Here's how the part is built. I have some questions about the finished solid (model axes, mm). Face numbers are marked on the shaded views. A direction names the side the tool comes from. Round coordinates to 2 decimals unless told otherwise and drop trailing zeros. Order: outer loops, then holes, each group sorted by start corner. A loop starts at its lowest first (then second) coordinate and runs counter-clockwise, first axis right, second up. Notation, with made-up numbers: (-6.75, -6.5) - (41.25, -6.5) arc R21 ccw to (41.25, 17.5) - close; hole circle Ø4 at (30, 83.5). An arc over 180 degrees is marked (long way). One line per item, written item: value.
Autodesk Inventor part; units mm, degrees
ref_plane "YZ Plane" through (0, 0, 0) normal (1, 0, 0) x (0, 1, 0)
ref_plane "XZ Plane" through (0, 0, 0) normal (0, 1, 0) x (-1, 0, 0)
ref_plane "XY Plane" through (0, 0, 0) normal (0, 0, 1) x (1, 0, 0)
sketch "Sketch1" plane through (0, 0, 0) normal (0, 0, 1) x (1, 0, 0)
  line L0 (0, 0) -> (8.89, 0)
  line L1 (8.89, 0) -> (8.89, 12.7)
  line L2 (8.89, 12.7) -> (0, 12.7)
  line L3 (0, 12.7) -> (0, 0)
  circle A0 centre (7.62, 1.27) radius 0.635
  circle A1 centre (1.27, 1.27) radius 0.635
  point P0 (4.445, 4.445)
  dimension "d0" = 8.89
  dimension "d1" = 12.7
  dimension "d18" = 1.27
  dimension "d19" = 1.27
  dimension "d20" = 1.27
  dimension "d21" = 1.27
  dimension "d22" = 1.27
  dimension "d23" = 1.27
  dimension "d26" = 4.445
extrude "Extrusion1" add sketch "Sketch1" along normal blind 2.54 contours L3 L2 L1 L0 | A0 | A1
sketch "Sketch2" plane through (0, 0, 2.54) normal (0, 0, 1) x (1, 0, 0)
  circle A0 centre (4.445, 10.16) radius 1.27
  line L0 (8.89, 12.7) -> (0, 12.7)
  line L1 (8.89, 0) -> (8.89, 12.7)
  point P0 (0, 0)
  dimension "d5" = 2.54
  dimension "d6" = 2.54
  dimension "d7" = 4.445
extrude "Extrusion2" add sketch "Sketch2" against normal blind 7.62
hole "Hole1" at (4.445, 4.445, 0) direction (0, 0, 1) diameter 4.9784 depth 19.05 tip angle 118
extrude "Extrusion3" cut sketch "Sketch1" along normal blind 5.08 contours A0 | A1
properties part number "Slider"
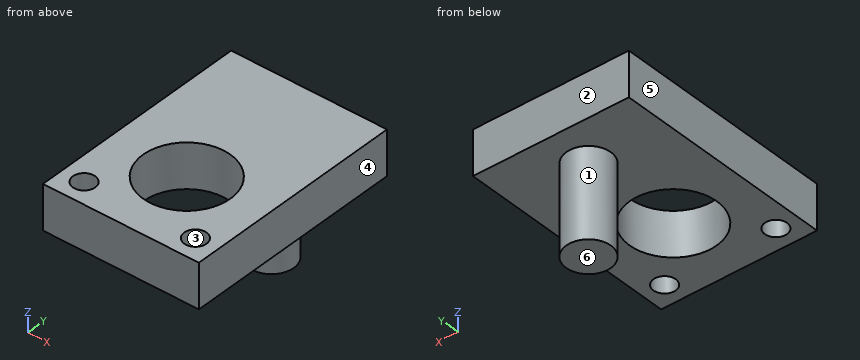
Q1. If we section it at B-B, the plane x = 1.27: Please give me the cut outline in (y, z) (3 decimals), then the cut area to 3 significant figures.
Results list:
outline: (0, 0) - (0.635, 0) - (0.635, 2.54) - (0, 2.54) - close; (1.905, 0) - (12.7, 0) - (12.7, 2.54) - (1.905, 2.54) - close
area: 29.0 mm²
Q2. If we section it at A-A, the plane y = 1.27: Please give me the cut outline in (x, z) (3 decimals), then the cut area to 3 significant figures.
Results list:
outline: (0, 0) - (0.635, 0) - (0.635, 2.54) - (0, 2.54) - close; (1.905, 0) - (6.985, 0) - (6.985, 2.54) - (1.905, 2.54) - close; (8.255, 0) - (8.89, 0) - (8.89, 2.54) - (8.255, 2.54) - close
area: 16.1 mm²
Q3. If I drill on line 1 along X through (y, z) = (1.27, 1.6) (3 decimals); line 2 along X through (y, z) = (0.75, 1.75); line 3 along Y through (x, z) = (1.27, 2) (3 decimals), over which ranges is the centre line in solid material (lowest first)?
Results list:
line 1: 0 to 0.635, 1.905 to 6.985, 8.255 to 8.89
line 2: 0 to 0.91, 1.63 to 7.26, 7.98 to 8.89
line 3: 0 to 0.635, 1.905 to 12.7
Q4. If we section it at C-C, the plane y = 6.5: Please give me the cut outline in (x, z), then the cut area to 3 significant figures.
Results list:
outline: (0, 0) - (3.04, 0) - (3.04, 2.54) - (0, 2.54) - close; (5.85, 0) - (8.89, 0) - (8.89, 2.54) - (5.85, 2.54) - close
area: 15.4 mm²
Q5. Will these pins go through, and if not, where does the flat tip stop? pin 1 (1.5 mm diameter, centred on y = 2.5, z = 0, fed in from -X); pin 2 (1.1 mm diameter, centred on x = 1.27, y = 1.27, fed in from -Z).
Results list:
pin 1: x = 0
pin 2: through
Q6. Which directions (+Z, -Z, +X, -X, +Y, -Y) give clear straight access to the entire face, cutting with the end or side of a thin tool? Please do the marked faces 1 and 2.
Results list:
face 1: -Z
face 2: +Z, -Z, +X, -X, +Y
Q7. If we section it at D-D, the plane z = 1.25: Please give me the cut outline in (x, y) (3 decimals), then the cut area to 3 significant figures.
Results list:
outline: (0, 0) - (8.89, 0) - (8.89, 12.7) - (0, 12.7) - close; hole circle Ø1.27 at (1.27, 1.27); hole circle Ø4.978 at (4.445, 4.445); hole circle Ø1.27 at (7.62, 1.27)
area: 90.9 mm²
Q8. We'd pull the mould along X, two halves only. Please class the marked faces 3, 4, 5 and 6: released by +X, released by -X, zero draft, split by the parting line, or undercut.
Results list:
face 3: undercut
face 4: released by +X
face 5: released by -X
face 6: zero draft
